```python
from build123d import *

# Parameters (mm, degrees)
SKETCH_W             = 36
SKETCH_H             = 36
PAD_DEPTH            = 22
PAD001_DEPTH         = 10
POCKET_DEPTH         = 10
SKETCH004_W          = 30
SKETCH004_H          = 30
POCKET001_DEPTH      = 20
PAD002_DEPTH         = 3
SKETCH006_R          = 0.5
POCKET002_DEPTH      = 18.001
POCKET002_DEPTH_BACK = 20.051
FILLET001_R          = 2.5
CHAMFER_SIZE2        = 4
CHAMFER_SIZE         = 0.8


with BuildPart() as part:
    # Sketch (on DatumPlane) → Pad (new body)
    with BuildSketch(Plane.XY):
        Rectangle(SKETCH_W, SKETCH_H)
    extrude(amount=PAD_DEPTH)

    # Sketch001 (on DatumPlane) → Pad001 (join)
    with BuildSketch(Plane.XY):
        Polygon((-1.7, 18), (1.7, 18), (2.6, 20.05), (-2.6, 20.05), align=None)
        Polygon((18, 1.7), (18, -1.7), (20.05, -2.6), (20.05, 2.6), align=None)
    extrude(amount=PAD001_DEPTH)

    # Sketch003 (on DatumPlane) → Pocket (cut)
    with BuildSketch(Plane.XY):
        Polygon((-2.05, -18), (2.05, -18), (3.1, -15.55), (-3.1, -15.55), align=None)
        Polygon((-18, 2.05), (-18, -2.05), (-15.55, -3.1), (-15.55, 3.1), align=None)
    extrude(amount=POCKET_DEPTH, mode=Mode.SUBTRACT)

    # Sketch004 (on DatumPlane) → Pocket001 (cut)
    with BuildSketch(Plane.XY.offset(22)):
        Rectangle(SKETCH004_W, SKETCH004_H)
    extrude(amount=-POCKET001_DEPTH, mode=Mode.SUBTRACT)

    # Sketch005 (on DatumPlane) → Pad002 (join)
    with BuildSketch(Plane.XY.offset(22)):
        Polygon((-18, 18), (-12, 18), (-12, 15), (-16.5, 15), (-16.5, -16.5), (16.5, -16.5), (16.5, 15), (12, 15), (12, 18), (18, 18), (18, -18), (-18, -18), align=None)
    extrude(amount=PAD002_DEPTH)

    # Sketch006 (on DatumPlane) → Pocket002 (cut, two sides)
    with BuildSketch(Plane.YZ) as pocket002_sk:
        with Locations((16.5, 23.5)):
            Circle(SKETCH006_R)
    extrude(amount=-POCKET002_DEPTH, mode=Mode.SUBTRACT)
    extrude(pocket002_sk.sketch, amount=POCKET002_DEPTH_BACK, mode=Mode.SUBTRACT)

    # Sketch007 (on DatumPlane) → AdditiveLoft section 0
    with BuildSketch(Plane(origin=(0, -16.5, 0), x_dir=(-1, 0, 0), z_dir=(0, -1, 0))):
        with BuildLine():
            ThreePointArc((-6, -22.75), (-6.75, -23.5), (-6, -24.25))
            Line((-6, -24.25), (6, -24.25))
            ThreePointArc((6, -24.25), (6.75, -23.5), (6, -22.75))
            Line((-6, -22.75), (6, -22.75))
        make_face()
    # Sketch008 (on DatumPlane) → AdditiveLoft section 1
    with BuildSketch(Plane.XZ.offset(15.7)):
        with BuildLine():
            ThreePointArc((-3.75, 24), (-4.25, 23.5), (-3.75, 23))
            Line((-3.75, 23), (3.75, 23))
            ThreePointArc((3.75, 23), (4.25, 23.5), (3.75, 24))
            Line((-3.75, 24), (3.75, 24))
        make_face()
    loft()

    # Fillet001
    fillet001_edges = [part.edges().sort_by_distance(p)[0] for p in [
        (-14.25, 15, 25),
        (14.25, 15, 25),
    ]]
    fillet(fillet001_edges, radius=FILLET001_R)

    # Chamfer
    chamfer_edges = [part.edges().sort_by_distance(p)[0] for p in [
        (15, 0, 22),
        (0, -15, 22),
        (-15, 0, 22),
    ]]
    chamfer_side = part.faces().sort_by_distance((-15.75, 14.543793, 22))[0]
    chamfer(chamfer_edges, length=CHAMFER_SIZE, length2=CHAMFER_SIZE2, reference=chamfer_side)


solid = part.part
```
Can you work these out from the model? Positions are in its coordinate system, mm. A direction names the side the tool comes from. Round coordinates to 2 decimals unless told otherwise and drop trailing zeros. Loops run counter-clockwise (first coordinate to the right, second up) from the corner with the lowest first, then second, coordinate; pieces in that order, holes last. Notation, with made-up numbers: M -5,66 L 51,66 A13 ccw 51,85 Z; hole C 18,77 d9. An arc over 180 degrees is marked long. Write item = value, one per line. Start each with the question number.
(1) If we mould it in two halves opening along X, with no side actions, what happens to faces 4 (the face through (1, 1, 0)), 5 (the face through (-2.156, 19.039, 4.93)), 6 (the face through (-0.2, -16.5, 22.5))? For each: released by +X, released by -X, zero draft, split by the parting line, or undercut.
(2) Suppose I cut it at C-C on y = 16.5. Write out the boundary of the cut face in (x, z).
(3) Suppose I cut it at A-A on z = 5.5. Write out the boundary of the cut face in (x, y), plus the area to 3 significant figures.
(4) I'm going to push flat-ended pins straight in: P1, Ø8, axis at x = 3, z = 5.5, coming from the +Y side; P2, Ø1.5, axis at x = -3.5, y = 16, coming from the +Z side; P3, Ø2, axis at x = 6, y = 5.5, coming from the +Z side; P4, Ø4, axis at x = -11, z = 6, coming from the +Y side. Where does each tip first touch, or does it pass through?
(5) I need wall thicknesses on line 1 along Y through (x, z) = (-3.5, 4.75); line 2 along X through (y, z) = (6.5, 23.5). Which ranges of each line are inside material? Lowest first, please.
(6) Which directions (+Z, -Z, +X, -X, +Y, -Y) give clear straight access to the entire face, cutting with the end or side of a thin tool? Please do faces 1 (the face through (0, 19, 10)), 2 (the face through (-15, 0, 10)), 3 (the face through (-2.58, -16.76, 4.93)).
(7) Suppose I cut it at B-B on y = 0.5. Write out the boundary of the cut face in (x, z), plus the area to 3 significant figures.
(8) Suppose I cut it at D-D on z = 17.5. Write out the boundary of the cut face in (x, y), plus the area to 3 significant figures.
Answer block:
q1.face_4 = zero draft
q1.face_5 = released by -X
q1.face_6 = undercut
q2.outline = M -18,0 L 18,0 L 18,23 L 12,23 L 12,22 L -12,22 L -12,23 L -18,23 Z; M -18,24 L -12,24 L -12,24.79 L -16.5,24.79 L -16.5,25 L -18,25 Z; M 12,24 L 18,24 L 18,25 L 16.5,25 L 16.5,24.79 L 12,24.79 Z
q3.outline = M -18,-18 L -2.05,-18 L -3.1,-15.55 L 3.1,-15.55 L 2.05,-18 L 18,-18 L 18,-1.7 L 20.05,-2.6 L 20.05,2.6 L 18,1.7 L 18,18 L 1.7,18 L 2.6,20.05 L -2.6,20.05 L -1.7,18 L -18,18 L -18,2.05 L -15.55,3.1 L -15.55,-3.1 L -18,-2.05 Z; hole M -15,-15 L 15,-15 L 15,15 L -15,15 Z
q3.area = 388 mm²
q4.P1 = 20.05
q4.P2 = 22
q4.P3 = 2
q4.P4 = 18
q5.line_1 = -18 to -15, 15 to 18
q5.line_2 = -18 to -16.5, 16.5 to 18
q6.face_1 = +Z, +X, -X, +Y
q6.face_2 = +Z
q6.face_3 = -Z
q7.outline = M -18,10 L -15.55,10 L -15.55,0 L 20.05,0 L 20.05,10 L 18,10 L 18,25 L 16.5,25 L 16.5,22 L 15.8,22 L 15,18 L 15,2 L -15,2 L -15,18 L -15.8,22 L -16.5,22 L -16.5,25 L -18,25 Z
q7.area = 194 mm²
q8.outline = M -18,-18 L 18,-18 L 18,18 L -18,18 Z; hole M -15,-15 L 15,-15 L 15,15 L -15,15 Z
q8.area = 396 mm²
